Source: CAD feature listing. Evaluate the final solid. Frame: model axes, mm. A direction names the side the tool comes from. Give positions to 0.01 mm unless a question says otherwise; leave off trailing zeros. Loops run counter-clockwise (first coordinate to the right, second up) from the corner with the lowest first, then second, coordinate; pieces in that order, holes last.
from build123d import *

# Parameters (mm, degrees)
F0_R     = 11.5
F1_DEPTH = 2
F2_R     = 11.5
F2_R_2   = 10.133636
F2_R_3   = 8.512332
F2_R_4   = 7.127684
F2_R_5   = 5.721488
F2_R_6   = 4.303126
F2_R_7   = 3.104156
F2_R_8   = 1.964911
F3_DEPTH = 1
F4_SIZE  = 0.5
F5_SIZE  = 0.5


with BuildPart() as f1:
    # F0 (on Front) → F1 (new body)
    with BuildSketch(Plane.XZ):
        Circle(F0_R)
    extrude(amount=F1_DEPTH)

    # F2 (on face) → F3 (join)
    with BuildSketch(Plane.XZ.offset(2)):
        Circle(F2_R)
        Circle(F2_R_2, mode=Mode.SUBTRACT)
        Circle(F2_R_3)
        Circle(F2_R_4, mode=Mode.SUBTRACT)
        Circle(F2_R_5)
        Circle(F2_R_6, mode=Mode.SUBTRACT)
        Circle(F2_R_7)
        Circle(F2_R_8, mode=Mode.SUBTRACT)
    extrude(amount=F3_DEPTH)

    # F4
    f4_edges = [f1.edges().sort_by_distance(p)[0] for p in [
        (-1.964911, -3, 0),
        (-4.303126, -3, 0),
        (-7.127684, -3, 0),
        (-10.133636, -3, 0),
    ]]
    chamfer(f4_edges, length=F4_SIZE)

    # F5
    f5_edges = [f1.edges().sort_by_distance(p)[0] for p in [
        (-3.104156, -3, 0),
        (-5.721488, -3, 0),
        (-8.512332, -3, 0),
    ]]
    chamfer(f5_edges, length=F5_SIZE)


solid = f1.part
1) Reachability of faces 5 (the flat face through (8, -3, -8)), 6 (the flat face through (0, -2, 6)) from +Z, -Z, +X, -X, +Y, -Y: full face, straight path, thin tool, end or side. Return the list, or none.
Checks:
face 5: +Z, -Z, +X, -X, -Y
face 6: -Y
2) Contact query for flat-ended pins moving along their axis: P1, Ø1.5, axis at y = -2.5, z = -2.5, coming from the -X side; P2, Ø1.2, axis at x = -0.5, z = 1, coming from the -Y side; P3, Ø1, axis at y = -2.5, z = -3.5, coming from the -X side. Output: stop coordinate, or through.
Checks:
P1: stops at x = -11.37
P2: stops at y = -2
P3: stops at x = -11.1
3) Cut plane A-A (y = -0.6). Return loops of the section in (x, z), and give its area (3 significant figures).
Checks:
outline: circle Ø23 at (0, 0)
area: 415 mm2
4) Ray query, probe 1 along Z at (x, y) = (5.25, -2.4); probe 2 along X at (y, z) = (-2.1, -7.25); probe 3 along Y at (x, z) = (2.5, -6.5). Return the intervals inside material, ascending.
Checks:
probe 1: z = -10.23 to -8.67, -6.7 to -4.82, -2.27 to 2.27, 4.82 to 6.7, 8.67 to 10.23
probe 2: x = -8.93 to -7.08, -4.46 to 4.46, 7.08 to 8.93
probe 3: y = -2 to 0
5) Pull-direction query (Z, two-part tool) for faces 1 (the cylindrical face through (-3.415, -2.246, -2.618)), 2 (the flat face through (0, 0, 0)), 3 (the cylindrical face through (1.874, -2.246, 0.59)), 4 (the cylindrical face through (-1.5, -1.5, 11.4)); classes: released by +Z, released by -Z, zero draft, split by the parting line, or undercut.
Checks:
face 1: undercut
face 2: zero draft
face 3: undercut
face 4: split by the parting line
